Input: part model. Units: mm. Frame: model coordinates. Coordinates: 2 decimals unless noted, no trailing zeros. Order: outer loops, then holes, each group sorted by start corner. A loop starts at its lowest first (then second) coordinate and runs counter-clockwise, first axis right, second up. Notation, with made-up numbers: (55, 9.25) -> (64, 9.25) arc R18 cw to (64, 20.25) -> close; hole circle Ø5 at (-20.75, 50). An arc over 180 degrees is marked (long way). Write each question's results on one line, items separated by ' | '.
```python
from build123d import *

# Parameters (mm, degrees)
F1_DEPTH = 20
F2_DEPTH = 30


with BuildPart() as f1:
    # F0 (on Top) → F1 (new body)
    with BuildSketch(Plane.XY):
        with BuildLine():
            Line((26.324494, 29.597269), (-41.123118, 29.597269))
            ThreePointArc((-41.123118, 29.597269), (-24.823095, 22.845579), (-18.071405, 6.545556))
            ThreePointArc((-18.071405, 6.545556), (-24.823095, -9.754467), (-41.123118, -16.506158))
            Line((-41.123118, -16.506158), (26.324494, -16.506158))
            Line((26.324494, -16.506158), (26.324494, 29.597269))
        make_face()
        with BuildLine():
            Line((-41.123118, 18.017708), (-41.123118, 29.597269))
            ThreePointArc((-41.123118, 29.597269), (-64.174832, 6.545556), (-41.123118, -16.506158))
            Line((-41.123118, -16.506158), (-41.123118, -4.926596))
            ThreePointArc((-41.123118, -4.926596), (-52.59527, 6.545556), (-41.123118, 18.017708))
        make_face()
    extrude(amount=F1_DEPTH)

    # F0 (on Top) → F2 (join)
    with BuildSketch(Plane.XY):
        with BuildLine():
            Line((-41.123118, 18.017708), (-41.123118, 29.597269))
            ThreePointArc((-41.123118, 29.597269), (-64.174832, 6.545556), (-41.123118, -16.506158))
            Line((-41.123118, -16.506158), (-41.123118, -4.926596))
            ThreePointArc((-41.123118, -4.926596), (-52.59527, 6.545556), (-41.123118, 18.017708))
        make_face()
        with BuildLine():
            ThreePointArc((-18.071405, 6.545556), (-24.823095, 22.845579), (-41.123118, 29.597269))
            Line((-41.123118, 29.597269), (-41.123118, 18.017708))
            ThreePointArc((-41.123118, 18.017708), (-33.011082, 14.657592), (-29.650966, 6.545556))
            ThreePointArc((-29.650966, 6.545556), (-33.011082, -1.566481), (-41.123118, -4.926596))
            Line((-41.123118, -4.926596), (-41.123118, -16.506158))
            ThreePointArc((-41.123118, -16.506158), (-24.823095, -9.754467), (-18.071405, 6.545556))
        make_face()
    extrude(amount=F2_DEPTH)


solid = f1.part
```
(1) Line query: line 1 along X through (y, z) = (6, 13.5); line 2 along Z through (x, y) = (1, 13.5); line 3 along X through (y, z) = (10, 18). Output: solid intervals per line, ascending. Write a range as from..to.
Return value:
line 1: -64.17..-52.58, -29.66..26.32 | line 2: 0..20 | line 3: -63.91..-52.06, -30.18..26.32
(2) Cut plane D-D, the plane x = -23. Return loops of the section in (y, z), plus the area to 3 significant figures.
Return value:
outline: (-16.51, 0) -> (29.6, 0) -> (29.6, 20) -> (20.79, 20) -> (20.79, 30) -> (-7.7, 30) -> (-7.7, 20) -> (-16.51, 20) -> close | area: 1,210 mm2
(3) Cut plane B-B, the plane y = -1. Return loops of the section in (x, z).
Return value:
outline: (-62.9, 0) -> (-49.76, 0) -> (-49.76, 30) -> (-62.9, 30) -> close; (-32.48, 0) -> (26.32, 0) -> (26.32, 20) -> (-19.34, 20) -> (-19.34, 30) -> (-32.48, 30) -> close
(4) Cut plane A-A, the plane z = 9.5. Return loops of the section in (x, y), plus the area to 3 significant figures.
Return value:
outline: (-41.12, -16.51) -> (26.32, -16.51) -> (26.32, 29.6) -> (-41.12, 29.6) arc R23.05 ccw to start; hole (-41.12, 18.02) arc R11.47 ccw (long way) to (-29.65, 6.55) arc R11.47 ccw to start | area: 3,530 mm2
(5) Pin query (flat end, axial travel): P1, Ø5, axis at x = -8, y = 21, coming from the +Z side. Return the tip coordinate at first contact, or that it passes through.
Return value:
P1: z = 20
(6) Cut plane C-C, the plane x = -47. Return loops of the section in (y, z), plus the area to 3 significant figures.
Return value:
outline: (-15.74, 0) -> (-3.31, 0) -> (-3.31, 30) -> (-15.74, 30) -> close; (16.4, 0) -> (28.84, 0) -> (28.84, 30) -> (16.4, 30) -> close | area: 746 mm2
